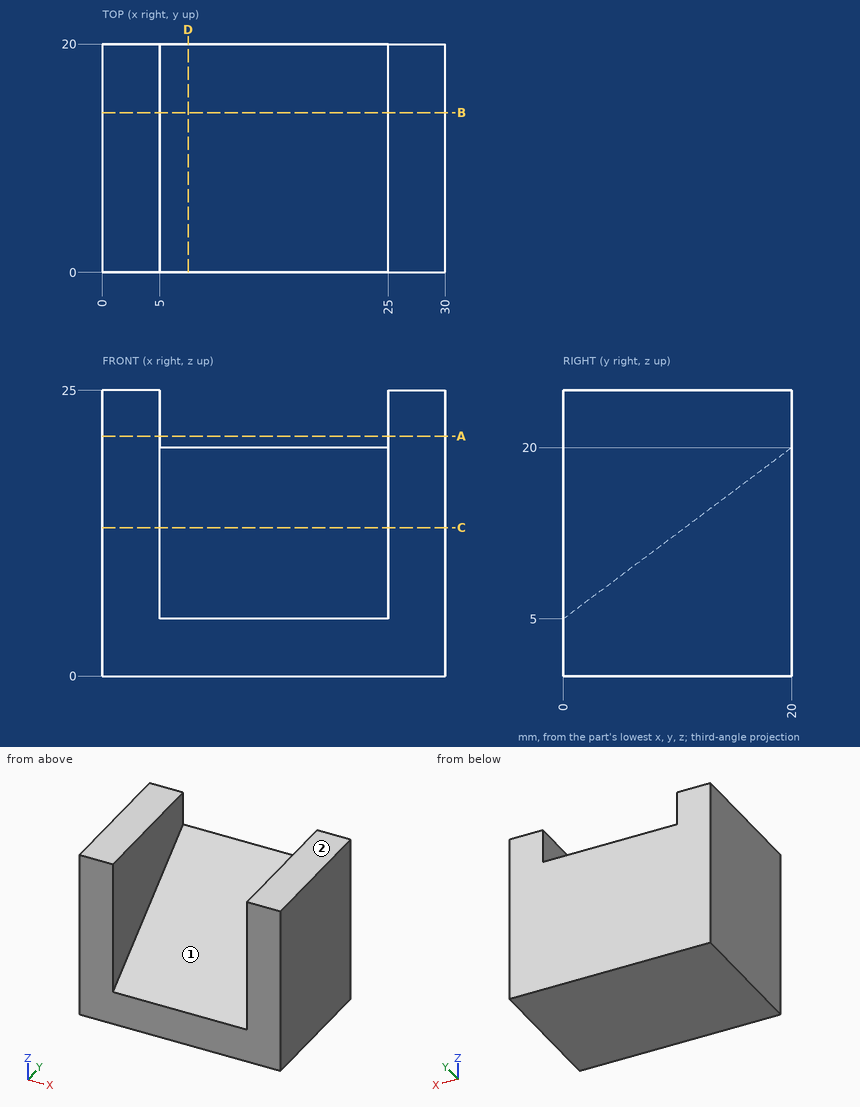
Part print with two shaded views. Sizes in mm from the minimum x, y, z corner. A direction names the side the tool comes from. Round coordinates to 2 decimals unless told otherwise and drop trailing zeros. Order: outer loops, then holes, each group sorted by start corner. A loop starts at its lowest first (then second) coordinate and runs counter-clockwise, first axis right, second up. Notation, with made-up numbers: (74.5, 83) -> (129.5, 83) arc R17 ccw to (129.5, 90) -> close; hole circle Ø10 at (81, 56). An arc over 180 degrees is marked (long way). One line per question, with ' | ' between items.
Q1. Slice it at D-D (x = 7.5). Write the cut outline in (y, z), then the cut area to 3 significant figures.
Completed:
outline: (0, 0) -> (20, 0) -> (20, 20) -> (0, 5) -> close | area: 250 mm^2
Q2. Which spindle directions (+Z, -Z, +X, -X, +Y, -Y) get a long thin tool onto all of the face, cutting with end or side? Do the marked faces 1 and 2. Say none if no direction does.
Completed:
face 1: +Z, -Y | face 2: +Z, +X, -X, +Y, -Y
Q3. Probe probe 1 along X at (y, z) = (5.5, 9.25); probe 2 along Y at (x, z) = (15.25, 12.25); probe 3 along Y at (x, z) = (7.25, 7). List the from-to ranges inside material, lowest first.
Completed:
probe 1: x = 0 to 5, 25 to 30 | probe 2: y = 9.67 to 20 | probe 3: y = 2.67 to 20
Q4. Slice it at B-B (y = 14). Write the cut outline in (x, z).
Completed:
outline: (0, 0) -> (30, 0) -> (30, 25) -> (25, 25) -> (25, 15.5) -> (5, 15.5) -> (5, 25) -> (0, 25) -> close
Q5. Slice it at C-C (z = 13). Write the cut outline in (x, y), then the cut area to 3 significant figures.
Completed:
outline: (0, 0) -> (5, 0) -> (5, 10.67) -> (25, 10.67) -> (25, 0) -> (30, 0) -> (30, 20) -> (0, 20) -> close | area: 387 mm^2
Q6. Drop a flat-ended pin along its axis: pin 1 (6 mm diameter, centred on x = 9, z = 20, fed in from -Y). Give the stop position or say it passes through.
Completed:
pin 1: stops at y = 16
Q7. Slice it at A-A (z = 21). Write the cut outline in (x, y).
Completed:
outline: (0, 0) -> (5, 0) -> (5, 20) -> (0, 20) -> close; (25, 0) -> (30, 0) -> (30, 20) -> (25, 20) -> close
